Here's how the part is built. I have some questions about the finished solid (model axes, mm). A direction names the side the tool comes from. Coordinates: 2 decimals unless noted, no trailing zeros. Write each loop counter-clockwise with the first axis right and the second up, starting at its lowest first coordinate (ties: lowest second). Pieces come first, ordered by that corner, then holes.
from build123d import *

# Parameters (mm, degrees)
SM_BASE_FLANGE_1_DEPTH      = 35
SKETCH_2_R                  = 1.6
CUT_EXTRUDE_1_DEPTH         = 74.952687578
PATTERN_LINEAR_1_COUNT      = 2
PATTERN_LINEAR_1_PITCH      = 20
CHAMFER_1_SIZE              = 3
SKETCH_3_R                  = 2.1
CUT_EXTRUDE_2_DEPTH         = 77.485292704
PATTERN_LINEAR_2_COUNT      = 2
PATTERN_LINEAR_2_PITCH      = 10
PATTERN_LINEAR_2_COUNT_DIR2 = 2
PATTERN_LINEAR_2_PITCH_DIR2 = 50
SKETCH_4_W                  = 20
SKETCH_4_H                  = 40
CUT_EXTRUDE_3_DEPTH         = 77.485292704
FILLET_1_R                  = 1


# Sheet-metal steps are written as plain solids
with BuildPart() as part:
    # Sketch 1 → 基材-凸緣1 (new body)
    with BuildSketch(Plane.XY):
        with BuildLine():
            Line((0, 65), (0, 3.7366))
            ThreePointArc((0, 3.7366), (1.094424801, 1.094424801), (3.7366, 0))
            Line((3.7366, 0), (20, 0))
            Line((20, 0), (20, 3))
            Line((20, 3), (3.7366, 3))
            ThreePointArc((3.7366, 3), (3.215745145, 3.215745145), (3, 3.7366))
            Line((3, 3.7366), (3, 65))
            Line((3, 65), (0, 65))
        make_face()
    extrude(amount=SM_BASE_FLANGE_1_DEPTH)

    # Sketch 2 → 除料-伸長1 (cut, through all)
    with BuildSketch(Plane(origin=(0, 3, 0), x_dir=(1, 0, 0), z_dir=(0, 1, 0))):
        with Locations(Location((13, -7.5, 0), (0, 0, 270))):
            Circle(SKETCH_2_R)
    cut_extrude_1 = extrude(amount=-CUT_EXTRUDE_1_DEPTH, mode=Mode.SUBTRACT)

    # 直線複製排列1: 除料-伸長1 ×2
    with Locations(*[(0, 0, i * PATTERN_LINEAR_1_PITCH) for i in range(1, PATTERN_LINEAR_1_COUNT)]):
        add(cut_extrude_1, mode=Mode.SUBTRACT)

    # 導角1
    chamfer_1_edges = [part.edges().sort_by_distance(p)[0] for p in [
        (20, 1.5, 35),
        (20, 1.5, 0),
        (1.5, 65, 35),
        (1.5, 65, 0),
    ]]
    chamfer(chamfer_1_edges, length=CHAMFER_1_SIZE)

    # 草圖3 → 除料-伸長2 (cut, through all)
    with BuildSketch(Plane.ZY):
        with Locations((12.5, 60)):
            Circle(SKETCH_3_R)
    cut_extrude_2 = extrude(amount=-CUT_EXTRUDE_2_DEPTH, mode=Mode.SUBTRACT)

    # 直線複製排列2: Cut-Extrude 2 2 × 2
    with Locations(*[(0, -j * PATTERN_LINEAR_2_PITCH_DIR2, i * PATTERN_LINEAR_2_PITCH) for i in range(PATTERN_LINEAR_2_COUNT) for j in range(PATTERN_LINEAR_2_COUNT_DIR2) if (i, j) != (0, 0)]):
        add(cut_extrude_2, mode=Mode.SUBTRACT)

    # 草圖4 → 除料-伸長3 (cut, through all)
    with BuildSketch(Plane.ZY):
        with Locations((17.5, 35)):
            Rectangle(SKETCH_4_W, SKETCH_4_H)
    extrude(amount=-CUT_EXTRUDE_3_DEPTH, mode=Mode.SUBTRACT)

    # 圓角1
    fillet_1_edges = [part.edges().sort_by_distance(p)[0] for p in [
        (1.5, 15, 7.5),
        (1.5, 55, 7.5),
        (1.5, 55, 27.5),
        (1.5, 15, 27.5),
    ]]
    fillet(fillet_1_edges, radius=FILLET_1_R)


solid = part.part
1. I want a section at B-B (y = 10). List the corners of the cut face in (x, z) for me, then the cut area to 3 significant figures.
2. I want a section at C-C (z = 12.5). List the corners of the cut face in (x, y) for me.
3. I want a section at D-D (y = 25). List the corners of the cut face in (x, z) for me.
4. If I drill on line 1 (Y direction, x = 7, z = 4); line 2 (Y direction, x = 1.9, z = 22.5), over which ranges is the centre line in solid material (lowest first)?
5. I want a section at A-A (x = 13). List the corners of the cut face in (y, z) for me, then the cut area to 3 significant figures.
6. For pin 1 Ø1.5 at (x, z) = (1, 13.5) entering from -Y; pin 2 Ø10 at (y, z) = (34, 12) entering from +X; pin 3 Ø8 at (x, z) = (11, 13.5) entering from +Y; pin 4 Ø2.5 at (y, z) = (60, 12.5) entering from +X, each with a flat end and sliding along its axis, tell me the tip position at first contact or that it passes through.
7. Thinking about a two-plate mould opening in X: for faces 4 (the face through (3, 34, 6)), 5 (the face through (14.08, 1.52, 6.32)), 6 (the face through (1.07, 1.12, 17.26)), 7 (the face through (1.479, 58.137, 23.469)), which applies, pulls with the +X half, pulls with the -X half, needs draft (parallel to the pull), parting line crosses it, or undercut?
8. On a 3-axis mill with a long thin cutter (end or side, diameter ignored), from which of +Z, -Z, +X, -X, +Y, -Y can I reach the whole of each face in a straight line? I mean faces 1 (the face through (1, 35, 7.5)), 2 (the face through (12, 3, 17)), 3 (the face through (12, 0, 17)). Say none if no direction works.
Response values:
1. outline: (0, 0) - (3, 0) - (3, 10.4) - (0, 10.4) - close; (0, 14.6) - (3, 14.6) - (3, 20.4) - (0, 20.4) - close; (0, 24.6) - (3, 24.6) - (3, 35) - (0, 35) - close
1. area: 79.8 mm2
2. outline: (0, 3.74) arc R3.74 ccw to (3.74, 0) - (20, 0) - (20, 3) - (3.74, 3) arc R0.74 cw to (3, 3.74) - (3, 7.9) - (0, 7.9) - close; (0, 12.1) - (3, 12.1) - (3, 15) - (0, 15) - close; (0, 55) - (3, 55) - (3, 57.9) - (0, 57.9) - close; (0, 62.1) - (3, 62.1) - (3, 65) - (0, 65) - close
3. outline: (0, 0) - (3, 0) - (3, 7.5) - (0, 7.5) - close; (0, 27.5) - (3, 27.5) - (3, 35) - (0, 35) - close
4. line 1: y = 0 to 3
4. line 2: y = 0.48 to 7.9, 12.1 to 15, 55 to 57.9, 62.1 to 65
5. outline: (0, 0) - (3, 0) - (3, 5.9) - (0, 5.9) - close; (0, 9.1) - (3, 9.1) - (3, 25.9) - (0, 25.9) - close; (0, 29.1) - (3, 29.1) - (3, 35) - (0, 35) - close
5. area: 85.8 mm2
6. pin 1: stops at y = 0.57
6. pin 2: stops at x = 3
6. pin 3: stops at y = 3
6. pin 4: passes through
7. face 4: pulls with the +X half
7. face 5: undercut
7. face 6: pulls with the -X half
7. face 7: needs draft
8. face 1: +X, -X
8. face 2: +Z, -Z, +X, +Y
8. face 3: +Z, -Z, +X, -X, -Y
